Check sheet for the drawn part. Datum: minimum x, y, z corner. Units: mm. Give positions to 0.01 mm unless a question says otherwise; leave off trailing zeros. Order: outer loops, then holes, each group sorted by start corner. A loop starts at its lowest first (then second) coordinate and runs counter-clockwise, first axis right, second up.
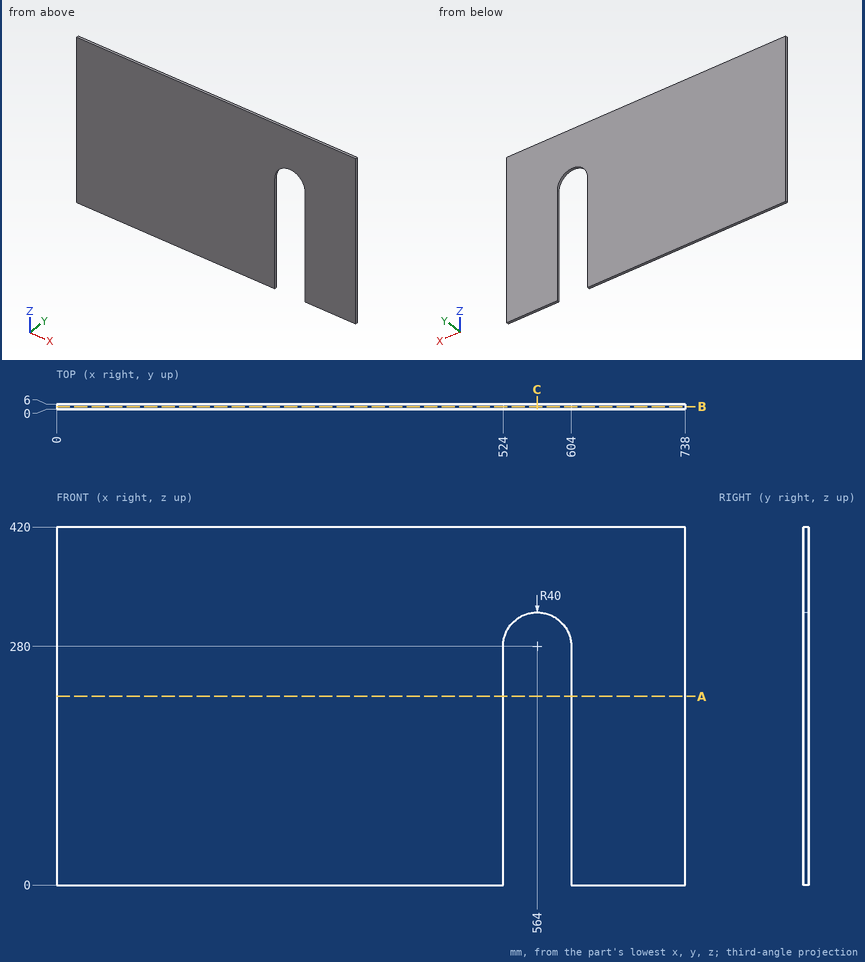
Item 1: Sectioned sample at A-A (z = 221.5). Enter the section's corners in (x, y).
Reported:
outline: (0, 0) - (524, 0) - (524, 6) - (0, 6) - close; (604, 0) - (738, 0) - (738, 6) - (604, 6) - close
Item 2: Sectioned sample at B-B (y = 3). Enter the section's corners in (x, z).
Reported:
outline: (0, 0) - (524, 0) - (524, 280) arc R40 cw to (604, 280) - (604, 0) - (738, 0) - (738, 420) - (0, 420) - close
Item 3: Scan lines: L1, parallel to X at y = 1.6, z = 228; L2, parallel to X at y = 4.85, z = 317; L3, parallel to Z at x = 557, y = 5.25. Record each from-to range of solid material in increasing order.
Reported:
L1: x = 0 to 524, 604 to 738
L2: x = 0 to 548.8, 579.2 to 738
L3: z = 319.38 to 420
Item 4: Sectioned sample at C-C (x = 564). Enter the section's corners in (y, z), and give its area (3 significant figures).
Reported:
outline: (0, 320) - (6, 320) - (6, 420) - (0, 420) - close
area: 600 mm2
